Work out the finished part from the listing and answer in its coordinate system (mm). A direction names the side the tool comes from. Round coordinates to 2 decimals unless told otherwise and drop trailing zeros. Order: outer loops, then holes, each group sorted by start corner. A loop starts at its lowest first (then second) coordinate and runs counter-clockwise, first axis right, second up. Notation, with made-up numbers: (83, 17) -> (109, 17) arc R17 cw to (109, 32) -> close; hole circle Ø8 at (60.25, 41.25). An arc over 180 degrees is marked (long way). Use one line per item in the form item = value.
```python
from build123d import *

# Parameters (mm, degrees)
SKETCH1_W           = 12.04
SKETCH1_H           = 7.58
SKETCH1_W_2         = 8.04
SKETCH1_H_2         = 3.58
BOSS_EXTRUDE1_DEPTH = 8
SKETCH1_2_W         = 12.04
SKETCH1_2_H         = 7.58
SKETCH1_2_W_2       = 8.04
SKETCH1_2_H_2       = 3.58
BOSS_EXTRUDE2_DEPTH = 2
EXTRUDE_THIN1_DEPTH = 12.04
SKETCH5_W           = 12.04
SKETCH5_H           = 7.58
SKETCH5_W_2         = 8.04
SKETCH5_H_2         = 3.58
BOSS_EXTRUDE4_DEPTH = 8
SKETCH5_4_W         = 12.04
SKETCH5_4_H         = 7.58
BOSS_EXTRUDE5_DEPTH = 2
CHAMFER1_SIZE       = 1.5
CHAMFER2_START      = -7
CHAMFER2_DEPTH      = 14


with BuildPart() as part:
    # Sketch1 → Boss-Extrude1 (new body)
    with BuildSketch(Plane.XY):
        Rectangle(SKETCH1_W, SKETCH1_H)
        Rectangle(SKETCH1_W_2, SKETCH1_H_2, mode=Mode.SUBTRACT)
    extrude(amount=BOSS_EXTRUDE1_DEPTH)

    # Sketch1<2> → Boss-Extrude2 (add)
    # profile 1 of 2: a face of its own
    with BuildSketch(Plane.XY):
        Rectangle(SKETCH1_2_W, SKETCH1_2_H)
        Rectangle(SKETCH1_2_W_2, SKETCH1_2_H_2, mode=Mode.SUBTRACT)
    # profile 2 of 2: a face of its own
    with BuildSketch(Plane.XY):
        Rectangle(SKETCH1_2_W_2, SKETCH1_2_H_2)
    extrude(amount=-BOSS_EXTRUDE2_DEPTH)

    # Sketch3 → Extrude-Thin1 (add)
    with BuildSketch(Plane(origin=(6.02, 9.81, 0), x_dir=(0, -1, 0), z_dir=(1, 0, 0))):
        with BuildLine():
            Line((6.02, 2.744137986), (6.52, 2.744137986))
            ThreePointArc((6.52, 2.744137986), (10.07949931, 2.557592532), (13.6, 2))
            Line((13.6, 2), (21.425180806, 0.336706473))
            ThreePointArc((21.425180806, 0.336706473), (22.120268588, 0.441550315), (22.574623539, 0.977927827))
            ThreePointArc((22.574623539, 0.977927827), (26.849152106, 14.317688881), (30.219561316, 27.914054616))
            Line((30.219561316, 27.914054616), (30.401286915, 28.769006338))
            Line((30.401286915, 28.769006338), (32.357582116, 28.353182957))
            Line((32.357582116, 28.353182957), (32.175856518, 27.498231234))
            ThreePointArc((32.175856518, 27.498231234), (28.773161162, 13.771621897), (24.457685624, 0.304075332))
            ThreePointArc((24.457685624, 0.304075332), (23.094620772, -1.305057203), (21.009357424, -1.619588728))
            Line((21.009357424, -1.619588728), (13.184176618, 0.043704799))
            ThreePointArc((13.184176618, 0.043704799), (9.870442383, 0.568548741), (6.52, 0.744137986))
            Line((6.52, 0.744137986), (6.02, 0.744137986))
            Line((6.02, 0.744137986), (6.02, 2.744137986))
        make_face()
    extrude(amount=-EXTRUDE_THIN1_DEPTH)



with BuildPart() as body_2:
    # Sketch5 → Boss-Extrude4 (new body)
    with BuildSketch(Plane(origin=(0, 484.189145571, -136.063399466), x_dir=(1, 0, 0), z_dir=(0, -0.20791169081775487, -0.9781476007338067))):
        with Locations((0, 517.847527624)):
            Rectangle(SKETCH5_W, SKETCH5_H)
        with Locations((0, 517.847527624)):
            Rectangle(SKETCH5_W_2, SKETCH5_H_2, mode=Mode.SUBTRACT)
    extrude(amount=BOSS_EXTRUDE4_DEPTH)


with BuildPart() as part_1:
    add(part.part)

    add(body_2.part)  # Boss-Extrude5 merges body 2
    # Sketch5<4> → Boss-Extrude5 (add)
    with BuildSketch(Plane(origin=(0, 484.189145571, -136.063399466), x_dir=(1, 0, 0), z_dir=(0, -0.20791169081775487, -0.9781476007338067))):
        with Locations((0, 517.847527624)):
            Rectangle(SKETCH5_4_W, SKETCH5_4_H)
    extrude(amount=-BOSS_EXTRUDE5_DEPTH)

    # Chamfer1
    chamfer1_edges = [part_1.edges().sort_by_distance(p)[0] for p in [
        (6.02, -26.673085599, -30.543301906),
        (-6.02, -26.673085599, -30.543301906),
        (6.02, 3.79, 2.627931007),
        (6.02, -3.79, 4.022340595),
        (-6.02, -3.79, 4.022340595),
        (-6.02, 3.79, 2.627931007),
        (6.02, -19.258726786, -32.119272522),
        (-6.02, -19.258726786, -32.119272522),
    ]]
    chamfer(chamfer1_edges, length=CHAMFER1_SIZE)

    # Chamfer2: read off the stored shape, not the designer's step
    # Chamfer2 outline → Chamfer2 (cut)
    with BuildSketch(Plane.YZ.offset(CHAMFER2_START)):
        with BuildLine():
            Line((3.79, -2.744137986), (3.79, -0.709020541))
            Line((3.79, -0.709020541), (1.696404781, -2.706829325))
            ThreePointArc((1.696404781, -2.706829325), (2.492984056, -2.734809543), (3.29, -2.744137986))
            Line((3.29, -2.744137986), (3.79, -2.744137986))
        make_face()
        Polygon((-25.633527145, -25.652563902), (-26.049350527, -27.608859104), (-23.677231944, -26.068387284), align=None)
        with BuildLine():
            ThreePointArc((-20.172493797, -26.813342374), (-20.172815684, -26.814817596), (-20.173137561, -26.81629282))
            Line((-20.173137561, -26.81629282), (-18.634991713, -29.18482972))
            Line((-18.634991713, -29.18482972), (-18.219168332, -27.228534519))
            Line((-18.219168332, -27.228534519), (-20.172493797, -26.813342374))
        make_face()
    extrude(amount=CHAMFER2_DEPTH, mode=Mode.SUBTRACT)


solid = part_1.part
```
Item 1: Consider line 1 along Y through (x, z) = (0.75, 3); line 2 along Z through (x, y) = (5.5, -1); line 3 along Z through (x, y) = (0, -2.5). Determine where each line is inside the solid, lowest interval first.
Findings:
line_1 = -3.79 to -1.79, 1.79 to 3.79
line_2 = -2.47 to 8
line_3 = -2.25 to 8
Item 2: Determine the mould class of faces 5 (the flat face through (-5.26, 3.05, 2.86)), 6 (the flat face through (0.084, -6.807, 0.686)), 7 (the flat face through (0, 0, 0)) for opening direction X: released by +X, released by -X, zero draft, split by the parting line, or undercut.
Findings:
face_5 = released by -X
face_6 = zero draft
face_7 = undercut
Item 3: The part is cut by section D-D, the plane z = -31.5. Give the vertices of the cut face in (x, y), and give its area (3 significant figures).
Findings:
outline = (-6.02, -25.34) -> (-4.52, -26.88) -> (4.52, -26.88) -> (6.02, -25.34) -> (6.02, -20.66) -> (4.52, -19.13) -> (-4.52, -19.13) -> (-6.02, -20.66) -> close; hole (-4.02, -24.83) -> (4.02, -24.83) -> (4.02, -21.17) -> (-4.02, -21.17) -> close
area = 59.3 mm^2
Item 4: The part is cut by section C-C, the plane y = 1. Give the vertices of the cut face in (x, z), and give its area (3 significant figures).
Findings:
outline = (-6.02, -2.67) -> (6.02, -2.67) -> (6.02, 8) -> (4.02, 8) -> (4.02, 0) -> (-4.02, 0) -> (-4.02, 8) -> (-6.02, 8) -> close
area = 64.1 mm^2
Item 5: The part is cut by section B-B, the plane z = 0.5. Give the vertices of the cut face in (x, y).
Findings:
outline = (-6.02, -14.21) -> (6.02, -14.21) -> (6.02, -5.93) -> (-6.02, -5.93) -> close; (-6.02, -2.29) -> (-4.52, -3.79) -> (4.52, -3.79) -> (6.02, -2.29) -> (6.02, 2.29) -> (4.52, 3.79) -> (-4.52, 3.79) -> (-6.02, 2.29) -> close; hole (-4.02, -1.79) -> (4.02, -1.79) -> (4.02, 1.79) -> (-4.02, 1.79) -> close
Item 6: For faces 1 (the flat face through (4.02, -23, -32)), 2 (the flat face through (4.02, 0, 4)), 3 (the flat face through (-0.056, -24.913, -31.882)), 4 (the flat face through (5.26, -3.05, 3.81)), determine the directions among +Z, -Z, +X, -X, +Y, -Y from which every point of the face is accessible in a straight line to the end or side of a thin tool.
Findings:
face_1 = none
face_2 = +Z
face_3 = -Z
face_4 = +Z, +X
Item 7: Flat-ended cylindrical pins translate along their axes: P1, Ø4, axis at x = 2, z = 6, coming from the -Y side; P2, Ø6, axis at x = 2, z = -30.5, coming from the -Y side; P3, Ø1.5, axis at x = 3, z = -22, coming from the -Y side. Find the tip coordinate at first contact, or state that the pin passes through.
Findings:
P1 = -3.79
P2 = -27.3
P3 = -21.3
